The listing builds one solid part. Answer for the finished solid, in the listing's coordinates (mm). A direction names the side the tool comes from. Give positions to 0.01 mm unless a question says otherwise; leave off trailing zeros. Loops run counter-clockwise (first coordinate to the right, second up) from the corner with the lowest first, then second, coordinate; pieces in that order, holes last. Notation, with made-up numbers: M 0,19 L 19,19 A15 cw 19,45 Z; hole C 58.25,-39.75 d9. An arc over 180 degrees is marked long. Use one line per item in the form item = value. Start each with the question number.
1. The mould has two halves that part along Y. Classify faces 3 (the face through (-16.216, -26.763, 2.274)), 4 (the face through (-26.763, 16.216, 2.274)), 5 (the face through (-20.956, 15.376, 2.218)), 6 (the face through (-12, 12, 4.5)): released by +Y, released by -Y, zero draft, split by the parting line, or undercut.
2. Straight lines are drawn through the part: line 1 (Y direction, x = 12, z = 3.5); line 2 (Y direction, x = 21, z = 1.25); line 3 (X direction, y = 0.5, z = 5.5). For each, find the intervals that lie inside material, in ascending order. Write a range as from..to.
3. Each of these flat-tipped pins is pushed along its axis until it touches: pin 1 Ø3.5 at (x, y) = (15.97, -22.39) entering from +Z; pin 2 Ø1.9 at (x, y) = (-15.97, -22.39) entering from -Z; pin 3 Ø2 at (x, z) = (-17.5, 1.5) entering from -Y; pin 4 Ø6.5 at (x, y) = (-20, 0) entering from -Z. Where does it stop, or does it pass through?
4. For faces 1 (the face through (10, 2, 2.5)), 2 (the face through (-27, -0.2, 3.8)), determine the directions among +Z, -Z, +X, -X, +Y, -Y from which every point of the face is accessible in a straight line to the end or side of a thin tool.
5. The part is cut by section C-C (z = 5.25). Write down the section's boundary in (x, y).
6. The part is cut by section D-D (x = -16.5). Give the number of separate pieces and of enclosed holes in the cut face, and give its area (3 significant figures).
7. The part is cut by section A-A (y = 0). Write down the section's boundary in (x, z), and give its area (3 significant figures).
8. The part is cut by section B-B (x = 0). Write down the section's boundary in (y, z).
from build123d import *

# Parameters (mm, degrees)
SKETCH_2_W               = 51
SKETCH_2_H               = 51
SKETCH_2_R               = 1.55
EXTRUDE_1_DEPTH          = 4.5
CUT_EXTRUDE_1_DEPTH      = 5
FILLET_1_R               = 4
SKETCH_5_R               = 13
CUT_EXTRUDE_2_DEPTH      = 2
CUT_EXTRUDE_3_DEPTH      = 37.14899722
CUT_EXTRUDE_3_DEPTH_BACK = 37.14899722
SKETCH_6_R               = 9.75
CUT_EXTRUDE_4_DEPTH      = 37.342124319
CUT_EXTRUDE_4_DEPTH_BACK = 2.3
SKETCH_8_W               = 28
SKETCH_8_H               = 8
EXTRUDE_START            = -4.5
EXTRUDE_2_DEPTH          = 4.5
CUT_EXTRUDE_7_DEPTH      = 39.448016854
CUT_EXTRUDE_7_DEPTH_BACK = 2.3
SKETCH_11_W              = 1.5
SKETCH_11_H              = 8
FILLET_3_R               = 1
FILLET_4_R               = 5
EXTRUDE_START_2          = 3
SKETCH_12_R              = 15
SKETCH_12_R_2            = 13
EXTRUDE_3_DEPTH          = 3
CUT_EXTRUDE_START        = -0.2
CUT_EXTRUDE_8_DEPTH      = 0.2
FILLET_5_R               = 2
CHAMFER_1_SIZE           = 0.5
CHAMFER_2_SIZE           = 0.5
CHAMFER_2_SIZE2          = 0.866025404


with BuildPart() as part:
    # 草图2 → 凸台-拉伸1 (new body)
    with BuildSketch(Plane.XY):
        Rectangle(SKETCH_2_W, SKETCH_2_H)
        with Locations((-22.388176755, 15.969331282)):
            Circle(SKETCH_2_R, mode=Mode.SUBTRACT)
        with Locations((-15.969331282, 22.388176755)):
            Circle(SKETCH_2_R, mode=Mode.SUBTRACT)
        with Locations(Location((15.969331282, 22.388176755, 0), (0, 0, 180))):
            Circle(SKETCH_2_R, mode=Mode.SUBTRACT)
        with Locations(Location((22.388176755, 15.969331282, 0), (0, 0, 180))):
            Circle(SKETCH_2_R, mode=Mode.SUBTRACT)
        with Locations((22.388176755, -15.969331282)):
            Circle(SKETCH_2_R, mode=Mode.SUBTRACT)
        with Locations((15.969331282, -22.388176755)):
            Circle(SKETCH_2_R, mode=Mode.SUBTRACT)
        with Locations(Location((-15.969331282, -22.388176755, 0), (0, 0, 180))):
            Circle(SKETCH_2_R, mode=Mode.SUBTRACT)
        with Locations(Location((-22.388176755, -15.969331282, 0), (0, 0, 180))):
            Circle(SKETCH_2_R, mode=Mode.SUBTRACT)
    extrude(amount=EXTRUDE_1_DEPTH)

    # 草图4 → 切除-拉伸1 (cut)
    with BuildSketch(Plane.XY.offset(4.5)):
        with BuildLine():
            Line((-25.5, -15.803480629), (-25.5, -25.5))
            Line((-25.5, -25.5), (-15.803480629, -25.5))
            ThreePointArc((-15.803480629, -25.5), (-21.213203436, -21.213203436), (-25.5, -15.803480629))
        make_face()
        with BuildLine():
            Line((15.803480629, -25.5), (25.5, -25.5))
            Line((25.5, -25.5), (25.5, -15.803480629))
            ThreePointArc((25.5, -15.803480629), (21.213203436, -21.213203436), (15.803480629, -25.5))
        make_face()
        with BuildLine():
            Line((25.5, 15.803480629), (25.5, 25.5))
            Line((25.5, 25.5), (15.803480629, 25.5))
            ThreePointArc((15.803480629, 25.5), (21.213203436, 21.213203436), (25.5, 15.803480629))
        make_face()
        with BuildLine():
            Line((-15.803480629, 25.5), (-25.5, 25.5))
            Line((-25.5, 25.5), (-25.5, 15.803480629))
            ThreePointArc((-25.5, 15.803480629), (-21.213203436, 21.213203436), (-15.803480629, 25.5))
        make_face()
    extrude(amount=-CUT_EXTRUDE_1_DEPTH, mode=Mode.SUBTRACT)

    # 圆角1
    fillet_1_edges = [part.edges().sort_by_distance(p)[0] for p in [
        (-15.803480629, -25.5, 2.25),
        (15.803480629, -25.5, 2.25),
        (-25.5, 15.803480629, 2.25),
        (15.803480629, 25.5, 2.25),
        (-15.803480629, 25.5, 2.25),
        (25.5, 15.803480629, 2.25),
        (25.5, -15.803480629, 2.25),
        (-25.5, -15.803480629, 2.25),
    ]]
    fillet(fillet_1_edges, radius=FILLET_1_R)

    # 草图5 → 切除-拉伸2 (cut)
    with BuildSketch(Plane.XY.offset(4.5)):
        Circle(SKETCH_5_R)
    extrude(amount=-CUT_EXTRUDE_2_DEPTH, mode=Mode.SUBTRACT)

    # 草图6 → 切除-拉伸3 (cut, two sides: drawn at the far end of the back side and taken through both)
    with BuildSketch(Plane.XY.offset(2.5).offset(-CUT_EXTRUDE_3_DEPTH_BACK)):
        Circle(SKETCH_6_R)
    extrude(amount=CUT_EXTRUDE_3_DEPTH + CUT_EXTRUDE_3_DEPTH_BACK, mode=Mode.SUBTRACT)

    # 草图8 → 切除-拉伸4 (cut, two sides: drawn at the far end of the back side and taken through both)
    with BuildSketch(Plane(origin=(0, 0, 0), x_dir=(-1, 0, 0), z_dir=(0, 0, -1)).offset(-CUT_EXTRUDE_4_DEPTH_BACK)):
        with Locations((22.891709622, 0)):
            Rectangle(SKETCH_8_W, SKETCH_8_H)
    extrude(amount=CUT_EXTRUDE_4_DEPTH + CUT_EXTRUDE_4_DEPTH_BACK, mode=Mode.SUBTRACT)

    # 草图9 → 凸台-拉伸2 (add)
    with BuildSketch(Plane(origin=(0, 0, 0), x_dir=(-1, 0, 0), z_dir=(0, 0, -1)).offset(EXTRUDE_START)):
        with BuildLine():
            ThreePointArc((-26.048076923, 17.712924338), (-26.09265794, 17.646326518), (-26.136263836, 17.579086183))
            Line((-26.136263836, 17.579086183), (-26.136263836, -17.579086183))
            ThreePointArc((-26.136263836, -17.579086183), (-26.09265794, -17.646326518), (-26.048076923, -17.712924338))
            ThreePointArc((-26.048076923, -17.712924338), (-22.273863607, -22.273863607), (-17.712924338, -26.048076923))
            ThreePointArc((-17.712924338, -26.048076923), (-16.238149632, -26.756635001), (-14.620191517, -27))
            Line((-14.620191517, -27), (14.620191517, -27))
            ThreePointArc((14.620191517, -27), (16.238149632, -26.756635001), (17.712924338, -26.048076923))
            ThreePointArc((17.712924338, -26.048076923), (22.273863607, -22.273863607), (26.048076923, -17.712924338))
            ThreePointArc((26.048076923, -17.712924338), (26.756635001, -16.238149632), (27, -14.620191517))
            Line((27, -14.620191517), (27, 14.620191517))
            ThreePointArc((27, 14.620191517), (26.756635001, 16.238149632), (26.048076923, 17.712924338))
            ThreePointArc((26.048076923, 17.712924338), (22.273863607, 22.273863607), (17.712924338, 26.048076923))
            ThreePointArc((17.712924338, 26.048076923), (16.238149632, 26.756635001), (14.620191517, 27))
            Line((14.620191517, 27), (-14.620191517, 27))
            ThreePointArc((-14.620191517, 27), (-16.238149632, 26.756635001), (-17.712924338, 26.048076923))
            ThreePointArc((-17.712924338, 26.048076923), (-22.273863607, 22.273863607), (-26.048076923, 17.712924338))
        make_face()
        with BuildLine():
            Line((25.5, 14.620191517), (25.5, 5))
            Line((25.5, 5), (25.5, 4))
            Line((25.5, 4), (25.5, -4))
            Line((25.5, -4), (25.5, -14.620191517))
            ThreePointArc((25.5, -14.620191517), (25.323007274, -15.796888328), (24.807692308, -16.869451751))
            ThreePointArc((24.807692308, -16.869451751), (21.213203436, -21.213203436), (16.869451751, -24.807692308))
            ThreePointArc((16.869451751, -24.807692308), (15.796888328, -25.323007274), (14.620191517, -25.5))
            Line((14.620191517, -25.5), (-14.620191517, -25.5))
            ThreePointArc((-14.620191517, -25.5), (-15.796888328, -25.323007274), (-16.869451751, -24.807692308))
            ThreePointArc((-16.869451751, -24.807692308), (-21.213203436, -21.213203436), (-24.807692308, -16.869451751))
            ThreePointArc((-24.807692308, -16.869451751), (-25.323007274, -15.796888328), (-25.5, -14.620191517))
            Line((-25.5, -14.620191517), (-25.5, 14.620191517))
            ThreePointArc((-25.5, 14.620191517), (-25.323007274, 15.796888328), (-24.807692308, 16.869451751))
            ThreePointArc((-24.807692308, 16.869451751), (-21.213203436, 21.213203436), (-16.869451751, 24.807692308))
            ThreePointArc((-16.869451751, 24.807692308), (-15.796888328, 25.323007274), (-14.620191517, 25.5))
            Line((-14.620191517, 25.5), (14.620191517, 25.5))
            ThreePointArc((14.620191517, 25.5), (15.796888328, 25.323007274), (16.869451751, 24.807692308))
            ThreePointArc((16.869451751, 24.807692308), (21.213203436, 21.213203436), (24.807692308, 16.869451751))
            ThreePointArc((24.807692308, 16.869451751), (25.323007274, 15.796888328), (25.5, 14.620191517))
        make_face(mode=Mode.SUBTRACT)
    extrude(amount=EXTRUDE_2_DEPTH)

    # 草图11 → 切除-拉伸7 (cut, two sides: drawn at the far end of the back side and taken through both)
    with BuildSketch(Plane(origin=(0, 0, 0), x_dir=(-1, 0, 0), z_dir=(0, 0, -1)).offset(-CUT_EXTRUDE_7_DEPTH_BACK)):
        with Locations((26.25, 0)):
            Rectangle(SKETCH_11_W, SKETCH_11_H)
    extrude(amount=CUT_EXTRUDE_7_DEPTH + CUT_EXTRUDE_7_DEPTH_BACK, mode=Mode.SUBTRACT)

    # 圆角3
    fillet_3_edges = [part.edges().sort_by_distance(p)[0] for p in [
        (-27, 4, 1.15),
        (-27, -4, 1.15),
        (-27, 0, 2.3),
    ]]
    fillet(fillet_3_edges, radius=FILLET_3_R)

    # 圆角4
    fillet_4_edges = [part.edges().sort_by_distance(p)[0] for p in [
        (26.136263836, 17.579086183, 2.25),
        (26.136263836, -17.579086183, 2.25),
    ]]
    fillet(fillet_4_edges, radius=FILLET_4_R)

    # 草图12 → 凸台-拉伸3 (add)
    with BuildSketch(Plane.XY.offset(4.5).offset(EXTRUDE_START_2)):
        Circle(SKETCH_12_R)
        Circle(SKETCH_12_R_2, mode=Mode.SUBTRACT)
    extrude(amount=-EXTRUDE_3_DEPTH)

    # 草图13 → 切除-拉伸8 (cut)
    with BuildSketch(Plane(origin=(0, 0, 2.3), x_dir=(-1, 0, 0), z_dir=(0, 0, -1)).offset(CUT_EXTRUDE_START)):
        with BuildLine():
            Line((8.891709622, 4), (12.369316877, 4))
            ThreePointArc((12.369316877, 4), (13, 0), (12.369316877, -4))
            Line((12.369316877, -4), (8.891709622, -4))
            ThreePointArc((8.891709622, -4), (9.75, 0), (8.891709622, 4))
        make_face()
    extrude(amount=CUT_EXTRUDE_8_DEPTH, mode=Mode.SUBTRACT)

    # 圆角5
    fillet_5_edges = [part.edges().sort_by_distance(p)[0] for p in [
        (-8.891709622, -4, 1.25),
        (-8.891709622, 4, 1.25),
    ]]
    fillet(fillet_5_edges, radius=FILLET_5_R)

    # 倒角1
    chamfer_1_edges = [part.edges().sort_by_distance(p)[0] for p in [
        (21.706505209, 22.827124909, 0),
        (16.238149632, -26.756635001, 0),
        (0, -27, 0),
        (-16.238149632, -26.756635001, 0),
        (-22.273863607, -22.273863607, 0),
        (-26.756635001, -16.238149632, 0),
        (-27, -9.810095759, 0),
        (-26.756635001, 16.238149632, 0),
        (-22.273863607, 22.273863607, 0),
        (-16.238149632, 26.756635001, 0),
        (0, 27, 0),
        (16.238149632, 26.756635001, 0),
        (16.238149632, -26.756635001, 4.5),
        (0, -27, 4.5),
        (-16.238149632, -26.756635001, 4.5),
        (-22.273863607, -22.273863607, 4.5),
        (-26.756635001, -16.238149632, 4.5),
        (-27, 0, 4.5),
        (-26.756635001, 16.238149632, 4.5),
        (-22.273863607, 22.273863607, 4.5),
        (-16.238149632, 26.756635001, 4.5),
        (0, 27, 4.5),
        (16.238149632, 26.756635001, 4.5),
        (21.706505209, 22.827124909, 4.5),
        (-27, 9.810095759, 0),
        (-18.051299338, 4, 0),
        (-26.707106781, 4.292893219, 0),
        (-26.707106781, -4.292893219, 0),
        (26.136263836, 0, 0),
        (21.706505209, -22.827124909, 0),
        (25.876510219, -17.575246148, 0),
        (25.876510219, 17.575246148, 0),
        (26.136263836, 0, 4.5),
        (21.706505209, -22.827124909, 4.5),
        (25.876510219, -17.575246148, 4.5),
        (25.876510219, 17.575246148, 4.5),
        (-15, 0, 7.5),
        (-18.051299338, -4, 0),
        (9.75, 0, 0),
        (-9.11329417, 4.26181802, 0),
        (-9.11329417, -4.26181802, 0),
    ]]
    chamfer(chamfer_1_edges, length=CHAMFER_1_SIZE)

    # 倒角2
    chamfer_2_edges = [part.edges().sort_by_distance(p)[0] for p in [
        (-13, 0, 7.5),
    ]]
    chamfer_2_side = [part.faces().sort_by_distance(p)[0] for p in [
        (-14.089878067, 0, 7.5),
    ]]
    chamfer(chamfer_2_edges, length=CHAMFER_2_SIZE, length2=CHAMFER_2_SIZE2, reference=chamfer_2_side[0])


solid = part.part
Derived:
q1.face_3 = released by -Y
q1.face_4 = released by +Y
q1.face_5 = undercut
q1.face_6 = zero draft
q2.line_1 = -27..-5, 5..27
q2.line_2 = -23.48..-16.66, -15.28..15.28, 16.66..23.48
q2.line_3 = -14.99..-12.99, 12.99..14.99
q3.pin_1 = 4.5
q3.pin_2 = through
q3.pin_3 = -26.67
q3.pin_4 = 2.3
q4.face_1 = +Z
q4.face_2 = +Z, -Z, -X, +Y, -Y
q5.outline = C 0,0 d30; hole C 0,0 d26
q6.separate_pieces = 3
q6.enclosed_holes = 0
q6.area = 195 mm2
q7.outline = M -27,3.3 A1 ccw -26,2.3 L -13,2.3 L -13,6.63 L -13.5,7.5 L -14.5,7.5 L -15,7 L -15,4.5 L -26.5,4.5 L -27,4 Z; M 9.75,0.5 L 10.25,0 L 25.64,0 L 26.14,0.5 L 26.14,4 L 25.64,4.5 L 15,4.5 L 15,7 L 14.5,7.5 L 13.5,7.5 L 13,6.63 L 13,2.5 L 9.75,2.5 Z
q7.area = 109 mm2
q8.outline = M -27,0.5 L -26.5,0 L -10.25,0 L -9.75,0.5 L -9.75,2.5 L -13,2.5 L -13,6.63 L -13.5,7.5 L -14.5,7.5 L -15,7 L -15,4.5 L -26.5,4.5 L -27,4 Z; M 9.75,0.5 L 10.25,0 L 26.5,0 L 27,0.5 L 27,4 L 26.5,4.5 L 15,4.5 L 15,7 L 14.5,7.5 L 13.5,7.5 L 13,6.63 L 13,2.5 L 9.75,2.5 Z
